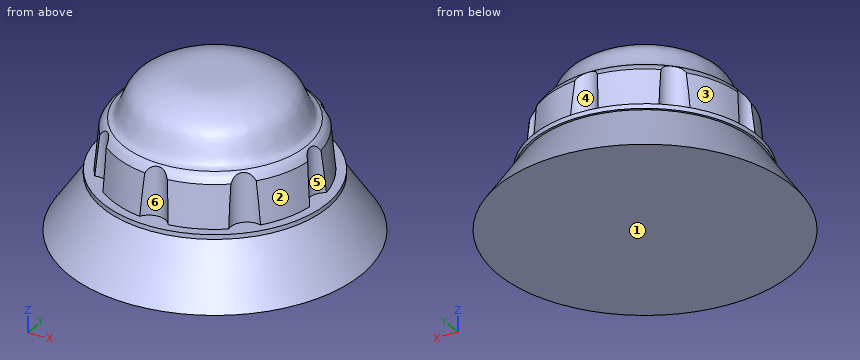
from build123d import *

# Parameters (mm, degrees)
F2_R     = 44.45
F3_DEPTH = 152.4


with BuildPart() as f1:
    # F0 (on Front) → F1 (revolve)
    with BuildSketch(Plane.XZ):
        Polygon((0, 152.4), (0, 0), (406.4, 0), (304.8, 152.4), align=None)
        with BuildLine():
            Line((0, 304.8), (0, 152.4))
            Line((0, 152.4), (304.8, 152.4))
            Line((304.8, 152.4), (311.15, 152.4))
            Line((311.15, 152.4), (311.15, 165.1))
            Line((311.15, 165.1), (285.75, 165.1))
            Line((285.75, 165.1), (274.5597064495, 280.7071506977))
            add(Edge.make_bspline(
                [(274.5597064495, 280.7071506977), (271.7412931371, 285.8037865906), (266.3064654877, 295.6317765268), (258.3550352472, 302.9362996616), (254, 304.8)],
                knots=[0, 0, 0, 0, 0.0771596923, 0.1487892593, 0.1487892593, 0.1487892593, 0.1487892593], degree=3))
            Line((254, 304.8), (0, 304.8))
        make_face()
        with BuildLine():
            Line((0, 432.1574568748), (0, 304.8))
            Line((0, 304.8), (254, 304.8))
            add(Edge.make_bspline(
                [(254, 304.8), (249.5133226892, 306.7200354412), (234.5546852881, 307.2114964849), (217.4700462275, 371.4836376253), (189.2452236448, 397.5288625798), (151.6517387873, 417.6984471616), (107.5702368284, 431.0904789048), (68.3418151338, 432.3167053391), (24.8362806494, 432.2153297824), (0, 432.1574568748)],
                knots=[0.1487892593, 0.1487892593, 0.1487892593, 0.1487892593, 0.222584013, 0.3675456115, 0.4848887913, 0.6047642941, 0.729359126, 0.8454975262, 1, 1, 1, 1], degree=3))
        make_face()
    revolve(axis=Axis((0, 0, 228.6), (0, 0, 1)))

    # F2 (on face) → F3 (cut)
    with BuildSketch(Plane.XY.offset(165.1)):
        with Locations((0, 304.8)):
            Circle(F2_R)
        with Locations((-215.5261469057, 215.5261469057)):
            Circle(F2_R)
        with Locations((-304.8, 0)):
            Circle(F2_R)
        with Locations((-215.5261469057, -215.5261469057)):
            Circle(F2_R)
        with Locations((0, -304.8)):
            Circle(F2_R)
        with Locations((215.5261469057, -215.5261469057)):
            Circle(F2_R)
        with Locations((304.8, 0)):
            Circle(F2_R)
        with Locations((215.5261469057, 215.5261469057)):
            Circle(F2_R)
    extrude(amount=F3_DEPTH, mode=Mode.SUBTRACT)


solid = f1.part
Here's how the part is built. I have some questions about the finished solid (model axes, mm). Face numbers are marked on the shaded views. A direction names the side the tool comes from. Give positions to 0.01 mm unless a question says otherwise; leave off trailing zeros. Order: outer loops, then holes, each group sorted by start corner. A loop starts at its lowest first (then second) coordinate and runs counter-clockwise, first axis right, second up. Notation, with made-up numbers: (15, 60) -> (74, 60) arc R26 ccw to (74, 93) -> close; hole circle Ø9 at (9.25, 26). An arc over 180 degrees is marked (long way). One line per item, written item: value. Start each with the question number.
1. We'd pull the mould along Z, two halves only. Please class the marked faces 1 and 2: released by +Z, released by -Z, zero draft, split by the parting line, or undercut.
2. Will these pins go through, and if not, where does the flat tip stop? pin 1 Ø2 at (x, y) = (52.5, 102.5) entering from +Z; pin 2 Ø10 at (y, z) = (37, 234) entering from -X; pin 3 Ø1 at (y, z) = (95.5, 148.5) entering from +X.
3. Imagine slicing it at C-C, the plane z = 186.5. List the corners of the cut face in (x, y) for me, plus the area to 3 significant figures.
4. Imagine slicing it at B-B, the plane z = 269.5. List the corners of the cut face in (x, y) for me, plus the area to 3 significant figures.
5. For the marked faces 3, 4, 5 and 6, which set-ups out of +Z, -Z, +X, -X, +Y, -Y let a thin tool reach every point of the face, with its end or its side?
6. I need wall thicknesses on probe 1 along Z at (x, y) = (-57.5, 7.5); probe 2 along Z at (x, y) = (3.5, 268); probe 3 along X at (y, z) = (163, 269.5). Which ranges of each line are inside material? Lowest first, please. Write a range as from..to.
7. Imagine slicing it at A-A, the plane z = 139.5. List the corners of the cut face in (x, y) for me, plus the area to 3 significant figures.
Values follow:
1. face 1: released by -Z
1. face 2: released by +Z
2. pin 1: stops at z = 428
2. pin 2: stops at x = -277.33
2. pin 3: stops at x = 292.58
3. outline: (-281.17, -37.65) arc R283.68 ccw to (-225.44, -172.2) arc R44.45 cw to (-172.2, -225.44) arc R283.68 ccw to (-37.65, -281.17) arc R44.45 cw to (37.65, -281.17) arc R283.68 ccw to (172.2, -225.44) arc R44.45 cw to (225.44, -172.2) arc R283.68 ccw to (281.17, -37.65) arc R44.45 cw to (281.17, 37.65) arc R283.68 ccw to (225.44, 172.2) arc R44.45 cw to (172.2, 225.44) arc R283.68 ccw to (37.65, 281.17) arc R44.45 cw to (-37.65, 281.17) arc R283.68 ccw to (-172.2, 225.44) arc R44.45 cw to (-225.44, 172.2) arc R283.68 ccw to (-281.17, 37.65) arc R44.45 cw to start
3. area: 243,000 mm2
4. outline: (-273.8, -31.85) arc R275.64 ccw to (-216.13, -171.08) arc R44.45 cw to (-171.08, -216.13) arc R275.64 ccw to (-31.85, -273.8) arc R44.45 cw to (31.85, -273.8) arc R275.64 ccw to (171.08, -216.13) arc R44.45 cw to (216.13, -171.08) arc R275.64 ccw to (273.8, -31.85) arc R44.45 cw to (273.8, 31.85) arc R275.64 ccw to (216.13, 171.08) arc R44.45 cw to (171.08, 216.13) arc R275.64 ccw to (31.85, 273.8) arc R44.45 cw to (-31.85, 273.8) arc R275.64 ccw to (-171.08, 216.13) arc R44.45 cw to (-216.13, 171.08) arc R275.64 ccw to (-273.8, 31.85) arc R44.45 cw to start
4. area: 233,000 mm2
5. face 3: +Z, -X, +Y
5. face 4: +Z, +Y
5. face 5: +Z, +X
5. face 6: +Z, -Y
6. probe 1: z = 0..432.13
6. probe 2: z = 0..165.1
6. probe 3: x = -222.29..222.29
7. outline: circle Ø626.8 at (0, 0)
7. area: 309,000 mm2
